```python
from build123d import *

# Parameters (mm, degrees)
SKETCH1_R           = 37.5
SKETCH1_R_2         = 32
BOSS_EXTRUDE1_DEPTH = 6.7
SKETCH2_R           = 37.5
SKETCH2_R_2         = 3.4
SKETCH2_R_3         = 1.5625
BOSS_EXTRUDE2_DEPTH = 12.85
CUT_EXTRUDE1_START  = -6.5
SKETCH3_R           = 5.5
SKETCH3_R_2         = 3.4
CUT_EXTRUDE1_DEPTH  = 6.5
SKETCH4_R           = 2.5
SKETCH4_R_2         = 1.5625
CUT_EXTRUDE2_DEPTH  = 2.5
FILLET1_R           = 5


with BuildPart() as part:
    # Sketch1 → Boss-Extrude1 (new body)
    with BuildSketch(Plane(origin=(0, 0, 0), x_dir=(1, 0, 0), z_dir=(0, 1, 0))):
        with Locations(Location((0, 0, 0), (0, 0, 270))):
            Circle(SKETCH1_R)
        with Locations(Location((0, 0, 0), (0, 0, 270))):
            Circle(SKETCH1_R_2, mode=Mode.SUBTRACT)
    extrude(amount=BOSS_EXTRUDE1_DEPTH)

    # Sketch2 → Boss-Extrude2 (add)
    with BuildSketch(Plane(origin=(0, 6.7, 0), x_dir=(1, 0, 0), z_dir=(0, 1, 0))):
        with Locations(Location((0, 0, 0), (0, 0, 270))):
            Circle(SKETCH2_R)
        with Locations(Location((-17.68, 17.68, 0), (0, 0, 90))):
            Circle(SKETCH2_R_2, mode=Mode.SUBTRACT)
        with Locations(Location((17.68, 17.68, 0), (0, 0, 90))):
            Circle(SKETCH2_R_2, mode=Mode.SUBTRACT)
        with Locations(Location((17.68, -17.68, 0), (0, 0, 90))):
            Circle(SKETCH2_R_2, mode=Mode.SUBTRACT)
        with Locations(Location((-17.68, -17.68, 0), (0, 0, 90))):
            Circle(SKETCH2_R_2, mode=Mode.SUBTRACT)
        with Locations(Location((0, 8, 0), (0, 0, 90))):
            Circle(SKETCH2_R_3, mode=Mode.SUBTRACT)
        with Locations(Location((8, 0, 0), (0, 0, 90))):
            Circle(SKETCH2_R_3, mode=Mode.SUBTRACT)
        with Locations(Location((-8, 0, 0), (0, 0, 90))):
            Circle(SKETCH2_R_3, mode=Mode.SUBTRACT)
        with Locations(Location((0, -8, 0), (0, 0, 90))):
            Circle(SKETCH2_R_3, mode=Mode.SUBTRACT)
    extrude(amount=BOSS_EXTRUDE2_DEPTH)

    # Sketch3 → Cut-Extrude1 (cut)
    # profile 1 of 4: a face of its own
    with BuildSketch(Plane(origin=(0, 19.55, 0), x_dir=(1, 0, 0), z_dir=(0, 1, 0)).offset(CUT_EXTRUDE1_START)):
        with Locations(Location((-17.68, 17.68, 0), (0, 0, 270))):
            Circle(SKETCH3_R)
        with Locations(Location((-17.68, 17.68, 0), (0, 0, 90))):
            Circle(SKETCH3_R_2, mode=Mode.SUBTRACT)
    # profile 2 of 4: a face of its own
    with BuildSketch(Plane(origin=(0, 19.55, 0), x_dir=(1, 0, 0), z_dir=(0, 1, 0)).offset(CUT_EXTRUDE1_START)):
        with Locations(Location((17.68, 17.68, 0), (0, 0, 270))):
            Circle(SKETCH3_R)
        with Locations(Location((17.68, 17.68, 0), (0, 0, 90))):
            Circle(SKETCH3_R_2, mode=Mode.SUBTRACT)
    # profile 3 of 4: a face of its own
    with BuildSketch(Plane(origin=(0, 19.55, 0), x_dir=(1, 0, 0), z_dir=(0, 1, 0)).offset(CUT_EXTRUDE1_START)):
        with Locations(Location((17.68, -17.68, 0), (0, 0, 270))):
            Circle(SKETCH3_R)
        with Locations(Location((17.68, -17.68, 0), (0, 0, 90))):
            Circle(SKETCH3_R_2, mode=Mode.SUBTRACT)
    # profile 4 of 4: a face of its own
    with BuildSketch(Plane(origin=(0, 19.55, 0), x_dir=(1, 0, 0), z_dir=(0, 1, 0)).offset(CUT_EXTRUDE1_START)):
        with Locations(Location((-17.68, -17.68, 0), (0, 0, 270))):
            Circle(SKETCH3_R)
        with Locations(Location((-17.68, -17.68, 0), (0, 0, 90))):
            Circle(SKETCH3_R_2, mode=Mode.SUBTRACT)
    extrude(amount=CUT_EXTRUDE1_DEPTH, mode=Mode.SUBTRACT)

    # Sketch4 → Cut-Extrude2 (cut)
    # profile 1 of 4: a face of its own
    with BuildSketch(Plane.XZ.offset(-6.7)):
        with Locations(Location((0, 8, 0), (0, 0, 270))):
            Circle(SKETCH4_R)
        with Locations(Location((0, 8, 0), (0, 0, 270))):
            Circle(SKETCH4_R_2, mode=Mode.SUBTRACT)
    # profile 2 of 4: a face of its own
    with BuildSketch(Plane.XZ.offset(-6.7)):
        with Locations(Location((8, 0, 0), (0, 0, 270))):
            Circle(SKETCH4_R)
        with Locations(Location((8, 0, 0), (0, 0, 270))):
            Circle(SKETCH4_R_2, mode=Mode.SUBTRACT)
    # profile 3 of 4: a face of its own
    with BuildSketch(Plane.XZ.offset(-6.7)):
        with Locations(Location((0, -8, 0), (0, 0, 270))):
            Circle(SKETCH4_R)
        with Locations(Location((0, -8, 0), (0, 0, 270))):
            Circle(SKETCH4_R_2, mode=Mode.SUBTRACT)
    # profile 4 of 4: a face of its own
    with BuildSketch(Plane.XZ.offset(-6.7)):
        with Locations(Location((-8, 0, 0), (0, 0, 270))):
            Circle(SKETCH4_R)
        with Locations(Location((-8, 0, 0), (0, 0, 270))):
            Circle(SKETCH4_R_2, mode=Mode.SUBTRACT)
    extrude(amount=-CUT_EXTRUDE2_DEPTH, mode=Mode.SUBTRACT)

    # Fillet1
    fillet1_edges = [part.edges().sort_by_distance(p)[0] for p in [
        (0, 19.55, -37.5),
    ]]
    fillet(fillet1_edges, radius=FILLET1_R)


solid = part.part
```
Model file for the job. Use its own axes, mm. A direction names the side the tool comes from. Round coordinates to 2 decimals unless told otherwise and drop trailing zeros. Write each loop counter-clockwise with the first axis right and the second up, starting at its lowest first coordinate (ties: lowest second). Pieces come first, ordered by that corner, then holes. Notation, with made-up numbers: (55, -38.5) -> (81, -38.5) arc R21 cw to (81, -9.5) -> close; hole circle Ø1 at (-22, 40). An arc over 180 degrees is marked (long way). Answer as CSV lines item,"result".
1. Drill centre lines: line 1 (X direction, y = 12.75, z = 0); line 2 (Z direction, x = 0.5, y = 1.5); line 3 (X direction, y = 17.5, z = 22). Where is each one in solid material? Low to high.
Resolved:
line 1,"-37.5 to -9.56, -6.44 to 6.44, 9.56 to 37.5"
line 2,"-37.5 to -32, 32 to 37.5"
line 3,"-29.17 to -21.08, -14.28 to 14.28, 21.08 to 29.17"
2. Slice it at B-B, the plane y = 12. State how many separate pieces and enclosed holes the cut face has, plus the area to 3 significant figures.
Resolved:
separate pieces,"1"
enclosed holes,"8"
area,"4,240 mm²"
3. Tool access for faces 3 (the face through (19.332, 16.254, 22.926)), 4 (the face through (-2, 9.2, -8)), 5 (the face through (6.45, 14.3, 0.2)): list every direction of +Z, -Z, +X, -X, +Y, -Y with a clear straight run to the whole face (end or side of a thin tool).
Resolved:
face 3,"+Y"
face 4,"-Y"
face 5,"+Y, -Y"
4. Slice it at A-A, the plane z = 0. List the corners of the cut face in (x, y).
Resolved:
outline,"(-37.5, 0) -> (-32, 0) -> (-32, 6.7) -> (-10.5, 6.7) -> (-10.5, 9.2) -> (-9.56, 9.2) -> (-9.56, 19.55) -> (-32.5, 19.55) arc R5 ccw to (-37.5, 14.55) -> close; (-6.44, 9.2) -> (-5.5, 9.2) -> (-5.5, 6.7) -> (5.5, 6.7) -> (5.5, 9.2) -> (6.44, 9.2) -> (6.44, 19.55) -> (-6.44, 19.55) -> close; (9.56, 9.2) -> (10.5, 9.2) -> (10.5, 6.7) -> (32, 6.7) -> (32, 0) -> (37.5, 0) -> (37.5, 14.55) arc R5 ccw to (32.5, 19.55) -> (9.56, 19.55) -> close"
5. Pin check, flat tips, straight feed: pin 1 Ø8 at (x, z) = (-17.68, -17.68) entering from +Y; pin 2 Ø3 at (x, z) = (0, 8) entering from +Y; pin 3 Ø8 at (y, z) = (10, -8.5) entering from -X; pin 4 Ø10 at (y, z) = (5, 14) entering from -X. Stop position of each tip, or through.
Resolved:
pin 1,"y = 13.05"
pin 2,"through"
pin 3,"x = -37.23"
pin 4,"x = -36.4"
6. Slice it at C-C, the plane y = 3.25. List the corners of the cut face in (x, z), plus the area to 3 significant figures.
Resolved:
outline,"circle Ø75 at (0, 0); hole circle Ø64 at (0, 0)"
area,"1,200 mm²"
7. Mould opens along Z. For faces 1 (the face through (17, 0, 28)), 2 (the face through (-9.55, 14.3, 0.2)) say: +Z half, -Z half, draft (parallel to the pull), parting line (faces both ways), or undercut.
Resolved:
face 1,"draft"
face 2,"undercut"
